Verification items for the finished model (mm, model axes). Round coordinates to 2 decimals unless told otherwise and drop trailing zeros. Order: outer loops, then holes, each group sorted by start corner. A loop starts at its lowest first (then second) coordinate and runs counter-clockwise, first axis right, second up. Notation, with made-up numbers: (-2.75, -16.5) -> (37.25, -16.5) arc R15 ccw to (37.25, -2.5) -> close; hole circle Ø7 at (-13, 2). An arc over 180 degrees is marked (long way). Put each result on its own line as item: value.
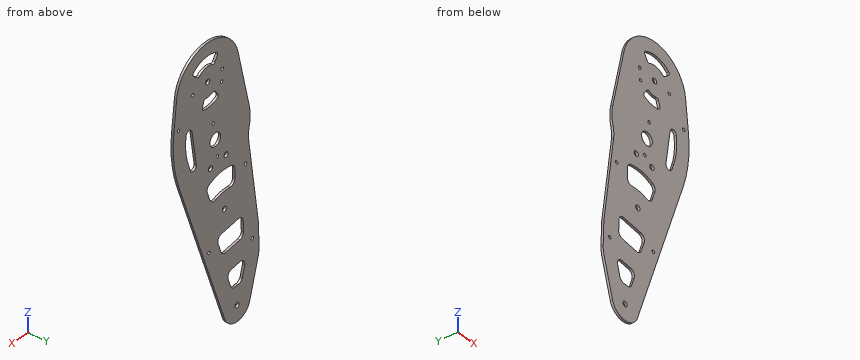
from build123d import *

# Parameters (mm, degrees)
SKETCH1_R           = 1.475
SKETCH1_R_2         = 2.455
SKETCH1_R_3         = 6.168108907
SKETCH1_R_4         = 2.425
BOSS_EXTRUDE1_DEPTH = 2.15


with BuildPart() as part:
    # Sketch1 → Boss-Extrude1 (new body)
    with BuildSketch(Plane(origin=(0, 0, 0), x_dir=(1, 0, 0), z_dir=(0, 1, 0))):
        with BuildLine():
            Line((-52.840792328, -53.480936505), (-39.943608053, -109.938847508))
            ThreePointArc((-39.943608053, -109.938847508), (-37.457286515, -117.158015126), (-33.49327647, -123.683718173))
            add(Edge.make_bspline(
                [(-33.49327647, -123.683718173), (-32.332703554, -125.083194688), (-31.130656762, -126.449768735), (-29.823601535, -127.783624049)],
                knots=[0.313138539, 0.313138539, 0.313138539, 0.313138539, 0.333887075, 0.333887075, 0.333887075, 0.333887075], degree=3))
            ThreePointArc((-29.823601535, -127.783624049), (7.100721182, -135.542158296), (30.379831892, -105.849003085))
            Line((30.379831892, -105.849003085), (33.615544776, -76.788996458))
            ThreePointArc((33.615544776, -76.788996458), (33.579883022, -49.913647939), (27.563931512, -23.720252642))
            Line((27.563931512, -23.720252642), (-24.684189405, 124.939833717))
            ThreePointArc((-24.684189405, 124.939833717), (-39.358339148, 134.957060264), (-53.29909759, 123.942036322))
            Line((-53.29909759, 123.942036322), (-62.855086574, 89.179051807))
            ThreePointArc((-62.855086574, 89.179051807), (-63.719958197, 84.755177464), (-63.912240207, 80.251657202))
            Line((-63.912240207, 80.251657202), (-63.229975042, 59.284277029))
            ThreePointArc((-63.229975042, 59.284277029), (-63.13826073, 57.721544859), (-62.965154571, 56.165724302))
            Line((-62.965154571, 56.165724302), (-52.006314121, -23.382858795))
            ThreePointArc((-52.006314121, -23.382858795), (-51.770839114, -29.123543867), (-52.634069461, -34.803838485))
            ThreePointArc((-52.634069461, -34.803838485), (-53.842880044, -44.130152103), (-52.840792328, -53.480936505))
        make_face()
        with Locations(Location((-21.173132912, -93.573319355, 0), (0, 0, 90))):
            Circle(SKETCH1_R, mode=Mode.SUBTRACT)
        with Locations(Location((-21.93278743, -104.537739321, 0), (0, 0, 90))):
            Circle(SKETCH1_R, mode=Mode.SUBTRACT)
        with Locations(Location((-5.125534576, -101.985044369, 0), (0, 0, 90))):
            Circle(SKETCH1_R_2, mode=Mode.SUBTRACT)
        with Locations(Location((11.681718278, -99.432349418, 0), (0, 0, 90))):
            Circle(SKETCH1_R, mode=Mode.SUBTRACT)
        with Locations(Location((28.194366713, -76.18652158, 0), (0, 0, 90))):
            Circle(SKETCH1_R, mode=Mode.SUBTRACT)
        with Locations(Location((-11.367714255, -60.885777039, 0), (0, 0, 90))):
            Circle(SKETCH1_R, mode=Mode.SUBTRACT)
        with Locations(Location((-13.845329944, -44.572855151, 0), (0, 0, 90))):
            Circle(SKETCH1_R_3, mode=Mode.SUBTRACT)
        with Locations(Location((-8.250860135, -21.470865896, 0), (0, 0, 90))):
            Circle(SKETCH1_R_4, mode=Mode.SUBTRACT)
        with Locations(Location((-16.322945632, -28.259933264, 0), (0, 0, 90))):
            Circle(SKETCH1_R, mode=Mode.SUBTRACT)
        with Locations(Location((-26.046774921, -24.173719374, 0), (0, 0, 90))):
            Circle(SKETCH1_R_4, mode=Mode.SUBTRACT)
        with Locations(Location((-56.366174752, 68.898827029, 0), (0, 0, 90))):
            Circle(SKETCH1_R, mode=Mode.SUBTRACT)
        with Locations(Location((-6.607589019, 54.284808215, 0), (0, 0, 90))):
            Circle(SKETCH1_R, mode=Mode.SUBTRACT)
        with Locations(Location((-24.303871319, 24.287448452, 0), (0, 0, 90))):
            Circle(SKETCH1_R_2, mode=Mode.SUBTRACT)
        with Locations(Location((-48.382600793, -3.644876674, 0), (0, 0, 90))):
            Circle(SKETCH1_R, mode=Mode.SUBTRACT)
        with Locations(Location((-38.835609181, 119.966171251, 0), (0, 0, 90))):
            Circle(SKETCH1_R_2, mode=Mode.SUBTRACT)
        with BuildLine():
            Line((-41.91710805, 82.298512317), (-32.399713849, 83.698520129))
            ThreePointArc((-32.399713849, 83.698520129), (-28.847563923, 86.060107453), (-28.410242809, 90.303174036))
            Line((-28.410242809, 90.303174036), (-31.382797644, 98.76089942))
            ThreePointArc((-31.382797644, 98.76089942), (-33.457293561, 101.347588782), (-36.693970949, 102.067598958))
            ThreePointArc((-36.693970949, 102.067598958), (-38.207418623, 101.950875498), (-39.725320718, 101.961896263))
            ThreePointArc((-39.725320718, 101.961896263), (-42.903984368, 101.018184144), (-44.793265793, 98.293278483))
            Line((-44.793265793, 98.293278483), (-47.465939738, 88.570567092))
            ThreePointArc((-47.465939738, 88.570567092), (-46.389618839, 83.932250043), (-41.91710805, 82.298512317))
        make_face(mode=Mode.SUBTRACT)
        with BuildLine():
            Line((-16.937854779, 51.629343597), (-20.390607974, 61.453363659))
            ThreePointArc((-20.390607974, 61.453363659), (-22.532582385, 64.081327612), (-25.858540532, 64.738785834))
            Line((-25.858540532, 64.738785834), (-41.906447635, 62.301420739))
            ThreePointArc((-41.906447635, 62.301420739), (-44.999859253, 60.55531199), (-46.153010078, 57.195500332))
            Line((-46.153010078, 57.195500332), (-45.817934871, 46.897965596))
            ThreePointArc((-45.817934871, 46.897965596), (-44.01778071, 43.216372089), (-40.069787164, 42.117266677))
            Line((-40.069787164, 42.117266677), (-20.904202072, 45.028146446))
            ThreePointArc((-20.904202072, 45.028146446), (-17.369143264, 47.396290594), (-16.937854779, 51.629343597))
        make_face(mode=Mode.SUBTRACT)
        with BuildLine():
            Line((-4.684973442, -1.328746966), (-7.754910594, 7.406057543))
            ThreePointArc((-7.754910594, 7.406057543), (-10.380057687, 10.289487703), (-14.277602246, 10.410785518))
            ThreePointArc((-14.277602246, 10.410785518), (-22.451748997, 8.304334218), (-30.891622317, 8.154833286))
            ThreePointArc((-30.891622317, 8.154833286), (-34.803601388, 6.83156599), (-36.385841207, 3.016971156))
            Line((-36.385841207, 3.016971156), (-36.0857593, -6.205149132))
            ThreePointArc((-36.0857593, -6.205149132), (-34.939447101, -9.23149884), (-32.179883099, -10.921951659))
            ThreePointArc((-32.179883099, -10.921951659), (-19.269492954, -11.43913062), (-7.004755403, -7.374421459))
            ThreePointArc((-7.004755403, -7.374421459), (-4.733969724, -4.777844919), (-4.684973442, -1.328746966))
        make_face(mode=Mode.SUBTRACT)
        with BuildLine():
            Line((19.844449525, -64.919654726), (19.667617674, -66.50778536))
            ThreePointArc((19.667617674, -66.50778536), (16.251850056, -69.619905943), (12.726728897, -66.632217245))
            Line((12.726728897, -66.632217245), (7.887886505, -33.893633842))
            ThreePointArc((7.887886505, -33.893633842), (10.510299936, -29.984172811), (14.652269896, -32.221363596))
            Line((14.652269896, -32.221363596), (16.818642893, -38.385282818))
            ThreePointArc((16.818642893, -38.385282818), (19.826618648, -51.481980466), (19.844449525, -64.919654726))
        make_face(mode=Mode.SUBTRACT)
        with BuildLine():
            Line((-0.653102394, -86.753585136), (0.966375004, -81.238240696))
            ThreePointArc((0.966375004, -81.238240696), (0.756700894, -79.636373516), (-0.56827267, -78.712043082))
            ThreePointArc((-0.56827267, -78.712043082), (-8.686544033, -78.538926638), (-16.387320245, -81.114648864))
            ThreePointArc((-16.387320245, -81.114648864), (-17.378099073, -82.390697064), (-17.102704245, -83.982582545))
            Line((-17.102704245, -83.982582545), (-13.91868529, -88.768369276))
            ThreePointArc((-13.91868529, -88.768369276), (-12.769636594, -89.592800652), (-11.362539974, -89.451099911))
            ThreePointArc((-11.362539974, -89.451099911), (-7.227753948, -88.143777313), (-2.891266968, -88.164478235))
            ThreePointArc((-2.891266968, -88.164478235), (-1.505550947, -87.882005033), (-0.653102394, -86.753585136))
        make_face(mode=Mode.SUBTRACT)
        with BuildLine():
            Line((6.78872402, -112.475537308), (11.102902912, -116.274167565))
            ThreePointArc((11.102902912, -116.274167565), (11.780924168, -117.740533437), (11.154170887, -119.22953378))
            ThreePointArc((11.154170887, -119.22953378), (-1.564525119, -125.4311621), (-15.551007519, -123.285531193))
            ThreePointArc((-15.551007519, -123.285531193), (-16.591599383, -122.049768162), (-16.379535287, -120.44821563))
            Line((-16.379535287, -120.44821563), (-13.387764062, -115.539953588))
            ThreePointArc((-13.387764062, -115.539953588), (-12.272305428, -114.670613587), (-10.860697091, -114.756415123))
            ThreePointArc((-10.860697091, -114.756415123), (-3.023315204, -115.826311425), (4.142973552, -112.477649245))
            ThreePointArc((4.142973552, -112.477649245), (5.465449668, -111.976593436), (6.78872402, -112.475537308))
        make_face(mode=Mode.SUBTRACT)
    extrude(amount=BOSS_EXTRUDE1_DEPTH)


solid = part.part
Item 1: Section check A-A on z = 45. Record the boundary of the cut face in (x, y).
Check sheet entries:
outline: (-53.84, 0) -> (-20, 0) -> (-20, 2.15) -> (-53.84, 2.15) -> close; (-7.69, 0) -> (9.53, 0) -> (9.53, 2.15) -> (-7.69, 2.15) -> close; (18.72, 0) -> (32.92, 0) -> (32.92, 2.15) -> (18.72, 2.15) -> close
Item 2: Material ranges on L1, parallel to X at y = 0.2, z = -55; L2, parallel to X at y = 0.6, z = 63; L3, parallel to X at y = 1.35, z = -87, recorded low to high. Write a range as [from, to].
Check sheet entries:
L1: x = [-62.8, -46.08], [-18.12, -7.9], [-5.32, -0.1]
L2: x = [-50.67, 12.19], [20.03, 34.35]
L3: x = [-63.37, -47.64], [-28.41, -11.35]
Item 3: Section check C-C on z = -73.5. Record the boundary of the cut face in (x, y), then the cut area to 3 significant figures.
Check sheet entries:
outline: (-63.69, 0) -> (-6.61, 0) -> (-6.61, 2.15) -> (-63.69, 2.15) -> close
area: 123 mm^2
Item 4: Section check B-B on y = 1.8. State how many separate pieces and enclosed holes the cut face has, then the cut area to 3 significant figures.
Check sheet entries:
separate pieces: 1
enclosed holes: 21
area: 15,200 mm^2
Item 5: Gauge pin test, flat ends, axial feed: pin 1 Ø4 at (x, z) = (-26.05, 24.17) entering from -Y; pin 2 Ø1 at (y, z) = (1.5, 22.5) entering from +X. Record the tip position at first contact, or that the pin passes through.
Check sheet entries:
pin 1: passes through
pin 2: stops at x = 27.31
